```python
from build123d import *

# Parameters (mm, degrees)
SKETCH1_R                 = 33.274
BOSS_EXTRUDE1_DEPTH       = 6.35
PLATEMTGSCREW_D           = 2.8702
PLATEMTGSCREW_DEPTH       = 10.1854
PLATEMTGSCREW_CSINK_D     = 7.7978
PLATEMTGSCREW_CSINK_ANGLE = 82
PLATEMTGSCREW_TIP         = 0.862295074
SHAFTBORE_D               = 26.19375
SHAFTBORE_DEPTH           = 6.35
SHAFTBORE_TIP             = 7.86939642


with BuildPart() as part:
    # Sketch1 → Boss-Extrude1 (new body)
    with BuildSketch(Plane(origin=(0, 0, 0), x_dir=(1, 0, 0), z_dir=(0, 1, 0))):
        Circle(SKETCH1_R)
    extrude(amount=BOSS_EXTRUDE1_DEPTH)

    # PlateMtgScrew
    with Locations(Plane(origin=(0, 6.35, 0), x_dir=(1, 0, 0), z_dir=(0, 1, 0))):
        with Locations((0, 30.226), (-30.226, 0), (0, -30.226), (30.226, 0)):
            CounterSinkHole(PLATEMTGSCREW_D / 2, PLATEMTGSCREW_CSINK_D / 2, depth=PLATEMTGSCREW_DEPTH, counter_sink_angle=PLATEMTGSCREW_CSINK_ANGLE)
            with Locations((0, 0, -(PLATEMTGSCREW_DEPTH + PLATEMTGSCREW_TIP / 2))):  # 118° drill point
                Cone(0, PLATEMTGSCREW_D / 2, PLATEMTGSCREW_TIP, mode=Mode.SUBTRACT)

    # ShaftBore
    with Locations(Plane(origin=(0, 6.35, 0), x_dir=(1, 0, 0), z_dir=(0, 1, 0))):
        with Locations((0, 0)):
            Hole(SHAFTBORE_D / 2, depth=SHAFTBORE_DEPTH)
            with Locations((0, 0, -(SHAFTBORE_DEPTH + SHAFTBORE_TIP / 2))):  # 118° drill point
                Cone(0, SHAFTBORE_D / 2, SHAFTBORE_TIP, mode=Mode.SUBTRACT)


solid = part.part
```
For this review, take the finished solid that the model builds, in its own axes (mm). Round coordinates to 2 decimals unless told otherwise and drop trailing zeros. Write each loop counter-clockwise with the first axis right and the second up, starting at its lowest first coordinate (ties: lowest second). Pieces come first, ordered by that corner, then holes. Notation, with made-up numbers: (-29.75, 5.5) - (23.25, 5.5) arc R12 ccw to (23.25, 15.5) - close; hole circle Ø7 at (58, 89). An arc over 180 degrees is marked (long way). Answer as a JSON object with one key per item and string values.
1. We need section A-A on z = 5.5. Give the boundary of the cut face in (x, y).
Response values:
{"outline": "(-32.82, 0) - (-11.89, 0) - (-11.89, 6.35) - (-32.82, 6.35) - close; (11.89, 0) - (32.82, 0) - (32.82, 6.35) - (11.89, 6.35) - close"}
2. We need section D-D on x = 25.5. Give the boundary of the cut face in (y, z), then the cut area to 3 significant figures.
Response values:
{"outline": "(0, -21.38) - (6.35, -21.38) - (6.35, 21.38) - (0, 21.38) - close", "area": "271 mm2"}
3. We need section C-C on y = 2. Give the boundary of the cut face in (x, z), then the cut area to 3 significant figures.
Response values:
{"outline": "circle Ø66.55 at (0, 0); hole circle Ø2.87 at (-30.23, 0); hole circle Ø26.19 at (0, 0); hole circle Ø2.87 at (0, -30.23); hole circle Ø2.87 at (0, 30.23); hole circle Ø2.87 at (30.23, 0)", "area": "2,910 mm2"}
4. For pin 1 Ø4.5 at (x, z) = (0, -30.226) entering from +Y; pin 2 Ø1 at (x, y) = (-24.5, 5.5) entering from -Z; pin 3 Ø3 at (x, y) = (20, 4) entering from -Z, all flat-tipped, find the tip position at first contact; note any pin that passes through.
Response values:
{"pin 1": "stops at y = 4.45", "pin 2": "stops at z = -23.05", "pin 3": "stops at z = -27.66"}
5. We need section B-B on x = 0. Give the boundary of the cut face in (y, z).
Response values:
{"outline": "(0, -33.27) - (5.37, -33.27) - (3.52, -31.66) - (0, -31.66) - close; (0, -28.79) - (3.52, -28.79) - (6.35, -26.33) - (6.35, -13.1) - (0, -13.1) - close; (0, 13.1) - (6.35, 13.1) - (6.35, 26.33) - (3.52, 28.79) - (0, 28.79) - close; (0, 31.66) - (3.52, 31.66) - (5.37, 33.27) - (0, 33.27) - close"}
6. To check wall thickness, follow line 1 along Z through (x, y) = (0, 0.9); line 2 along Z through (x, y) = (1, 3.25). State the ranges of each line that lie inside material, in increasing order.
Response values:
{"line 1": "z = -33.27 to -31.66, -28.79 to -13.1, 13.1 to 28.79, 31.66 to 33.27", "line 2": "z = -33.26 to -31.26, -29.2 to -13.06, 13.06 to 29.2, 31.26 to 33.26"}
7. Draft analysis for pull direction Z (two halves, no side actions). For faces 1 (the face through (-28.792, 1.733, -0.063)), 2 (the face through (28.743, 3.653, -0.467)), 3 (the face through (31.74, 3.13, -9.99)), 4 (the face through (14, 0, 0)), state which applies: +Z half, -Z half, draft (parallel to the pull), parting line (faces both ways), or undercut.
Response values:
{"face 1": "undercut", "face 2": "undercut", "face 3": "parting line", "face 4": "draft"}
